The model under review builds one solid part; all positions refer to its coordinate system, in mm. A direction names the side the tool comes from. Round coordinates to 2 decimals unless told otherwise and drop trailing zeros. Order: outer loops, then holes, each group sorted by start corner. A loop starts at its lowest first (then second) coordinate and runs counter-clockwise, first axis right, second up.
1) Consider section D-D (y = 10.5). Give the boundary of the cut face in (x, z), then the cut area to 3 significant figures.
2) To check wall thickness, follow L1, parallel to X at y = 14.5, z = 0.95; L2, parallel to X at y = 27.5, z = 1.1; L3, parallel to Y at x = 10, z = 1.45. State the ranges of each line that lie inside material, in increasing order.
3) Machinability: for faces 4 (the face through (12, 2, 2)), 5 (the face through (25.264, 21.054, 0.986)), which of the approach directions +Z, -Z, +X, -X, +Y, -Y give a long, thin tool a straight path to every point of the face, cutting with its end or side? Answer none if there is none.
4) Clearance check with flat-ended pins moving along their axes: P1, Ø1, axis at x = 28, z = 1.5, coming from the -Y side; P2, Ø2.5, axis at x = 19.52, y = 36.04, coming from the +Z side. State where each tip first meets the part, or that it passes through.
5) Consider section A-A (y = 0). Give the boundary of the cut face in (x, z), then the cut area to 3 significant figures.
6) Mouldability with a two-part tool opening along X and no side actions: class faces 1 (the face through (12, 2, 0)), 2 (the face through (19.6, 40, 1)), 3 (the face through (13.615, 20.741, 0.986)) as pulls with the +X half, pulls with the -X half, needs draft (parallel to the pull), parting line crosses it, or undercut.
7) Consider section B-B (z = 0.3). Give the boundary of the cut face in (x, y).
8) Consider section C-C (x = 0). Give the boundary of the cut face in (y, z), then the cut area to 3 significant figures.
from build123d import *

# Parameters (mm, degrees)
BOSS_EXTRUDE1_DEPTH = 2
SKETCH2_R           = 2
CUT_EXTRUDE1_DEPTH  = 2


with BuildPart() as part:
    # Sketch1 → Boss-Extrude1 (new body)
    with BuildSketch(Plane.XY):
        with BuildLine():
            Line((19.521264396, 32.085798574), (31.169759249, 9.709248155))
            ThreePointArc((31.169759249, 9.709248155), (44.814386457, -11.087635415), (35.604813415, 12.017991221))
            Line((35.604813415, 12.017991221), (21.738791479, 38.654371533))
            ThreePointArc((21.738791479, 38.654371533), (19.521264396, 40), (17.303737313, 38.654371533))
            Line((17.303737313, 38.654371533), (3.437715376, 12.017991221))
            ThreePointArc((3.437715376, 12.017991221), (-5.771857665, -11.087635415), (7.872769542, 9.709248155))
            Line((7.872769542, 9.709248155), (19.521264396, 32.085798574))
        make_face()
    extrude(amount=BOSS_EXTRUDE1_DEPTH)

    # Sketch2 → Cut-Extrude1 (cut)
    with BuildSketch(Plane.XY.offset(2)):
        with Locations((19.521264396, 36.042899287)):
            Circle(SKETCH2_R)
    extrude(amount=-CUT_EXTRUDE1_DEPTH, mode=Mode.SUBTRACT)


solid = part.part
Answer below:
1. outline: (-6.78, 0) - (8.28, 0) - (8.28, 2) - (-6.78, 2) - close; (30.76, 0) - (45.82, 0) - (45.82, 2) - (30.76, 2) - close
1. area: 60.3 mm2
2. L1: x = 4.73 to 10.37, 28.68 to 34.31
2. L2: x = 11.5 to 17.13, 21.91 to 27.55
2. L3: y = -7.5 to 7.5, 13.8 to 24.62
3. face 4: +Z, +X, -X, +Y, -Y
3. face 5: +Z, -Z
4. P1: stops at y = -6.72
4. P2: passes through
5. outline: (-12.5, 0) - (12.5, 0) - (12.5, 2) - (-12.5, 2) - close; (26.54, 0) - (51.54, 0) - (51.54, 2) - (26.54, 2) - close
5. area: 100 mm2
6. face 1: needs draft
6. face 2: parting line crosses it
6. face 3: undercut
7. outline: (3.44, 12.02) arc R12.5 ccw (long way) to (7.87, 9.71) - (19.52, 32.09) - (31.17, 9.71) arc R12.5 ccw (long way) to (35.6, 12.02) - (21.74, 38.65) arc R2.5 ccw to (17.3, 38.65) - close; hole circle Ø4 at (19.52, 36.04)
8. outline: (-12.5, 0) - (12.5, 0) - (12.5, 2) - (-12.5, 2) - close
8. area: 50.0 mm2
